from build123d import *

# Parameters (mm, degrees)
BOSS_EXTRUDE1_DEPTH = 26.5
SKETCH2_W           = 0.4
SKETCH2_H           = 5
SKETCH2_W_2         = 0.5
SKETCH2_H_2         = 1
BOSS_EXTRUDE2_DEPTH = 3.5
FILLET1_R           = 1


with BuildPart() as part:
    # Sketch1 → Boss-Extrude1 (new body)
    with BuildSketch(Plane(origin=(0, 0, 0), x_dir=(1, 0, 0), z_dir=(0, 1, 0))):
        with BuildLine():
            Line((-16, -7), (16, -7))
            ThreePointArc((16, -7), (16.707106781, -6.707106781), (17, -6))
            Line((17, -6), (17, 6))
            ThreePointArc((17, 6), (16.707106781, 6.707106781), (16, 7))
            Line((16, 7), (-16, 7))
            ThreePointArc((-16, 7), (-16.707106781, 6.707106781), (-17, 6))
            Line((-17, 6), (-17, -6))
            ThreePointArc((-17, -6), (-16.707106781, -6.707106781), (-16, -7))
        make_face()
    extrude(amount=BOSS_EXTRUDE1_DEPTH)

    # Sketch2 → Boss-Extrude2 (add)
    with BuildSketch(Plane.XZ):
        with Locations((-15, 0)):
            Rectangle(SKETCH2_W, SKETCH2_H)
        with Locations((15, 0)):
            Rectangle(SKETCH2_W, SKETCH2_H)
        with Locations((-2, 3.3)):
            Rectangle(SKETCH2_W_2, SKETCH2_H_2)
        with Locations((2, 3.3)):
            Rectangle(SKETCH2_W_2, SKETCH2_H_2)
    extrude(amount=BOSS_EXTRUDE2_DEPTH)

    # Fillet1
    fillet1_edges = [part.edges().sort_by_distance(p)[0] for p in [
        (-16.707106781, 26.5, -6.707106781),
        (-17, 26.5, 0),
        (-16.707106781, 26.5, 6.707106781),
        (0, 26.5, 7),
        (16.707106781, 26.5, 6.707106781),
        (17, 26.5, 0),
        (16.707106781, 26.5, -6.707106781),
        (0, 26.5, -7),
    ]]
    fillet(fillet1_edges, radius=FILLET1_R)


solid = part.part
Work out the finished part from the listing and answer in its coordinate system (mm). A direction names the side the tool comes from. Give positions to 0.01 mm unless a question says otherwise; leave off trailing zeros. Order: outer loops, then holes, each group sorted by start corner. A loop starts at its lowest first (then second) coordinate and runs counter-clockwise, first axis right, second up. Notation, with made-up numbers: (68, 84) -> (76, 84) arc R16 cw to (76, 107) -> close; hole circle Ø7 at (17, 73). An arc over 180 degrees is marked (long way). Answer as a JSON object with one key per item and string values. Group by question number.
1. Flat-ended cylindrical pins translate along their axes: pin 1 Ø4 at (x, z) = (1, -0.5) entering from -Y; pin 2 Ø1 at (y, z) = (-2.5, 0) entering from +X; pin 3 Ø1 at (y, z) = (-2, -0.5) entering from -X. Find the tip coordinate at first contact, or state that the pin passes through.
2. Section B-B on z = -5.25 is taken. Determine the outline of the cut face in (x, y).
3. A tool of negligible diameter and unlimited length cuts with its end or side. For faces 1 (the flat face through (2.25, -2, 3)), 2 (the flat face through (-17, 13, 0)), 3 (the flat face through (-15.2, -2, 0)), 4 (the flat face through (14.8, -2, 0)), from which of +Z, -Z, +X, -X, +Y, -Y can it reach the whole face along a straight path? Write none if from no direction.
4. Section A-A on x = -4 is taken. Determine the outline of the cut face in (y, z).
5. Consider line 1 along Y through (x, z) = (11.5, 3.25); line 2 along Y through (x, z) = (8.5, 6.75). Determine where each line is inside the solid, lowest interval first. Write a range as [from, to].
Result sheet:
{
 "1": {"pin 1": "stops at y = 0", "pin 2": "stops at x = 15.2", "pin 3": "stops at x = -15.2"},
 "2": {"outline": "(-17, 0) -> (17, 0) -> (17, 25.5) arc R1 ccw to (16, 26.5) -> (-16, 26.5) arc R1 ccw to (-17, 25.5) -> close"},
 "3": {"face 1": "+Z, -Z, +X, -Y", "face 2": "+Z, -Z, -X, +Y, -Y", "face 3": "+Z, -Z, -X, -Y", "face 4": "+Z, -Z, -Y"},
 "4": {"outline": "(0, -7) -> (25.5, -7) arc R1 ccw to (26.5, -6) -> (26.5, 6) arc R1 ccw to (25.5, 7) -> (0, 7) -> close"},
 "5": {"line 1": "y = [0, 26.5]", "line 2": "y = [0, 26.16]"}
}
